from build123d import *

# Parameters (mm, degrees)
PAD_DEPTH = 15
FILLET_R  = 1


with BuildPart() as part:
    # Sketch → Pad (new body)
    with BuildSketch(Plane.XY):
        with BuildLine():
            ThreePointArc((17.433407, 1.525225), (-17.5, 0), (17.433407, -1.525225))
            Line((17.433407, -1.525225), (25.402965, -2.222471))
            ThreePointArc((25.402965, 2.222471), (-25.5, 0), (25.402965, -2.222471))
            Line((17.433407, 1.525225), (25.402965, 2.222471))
        make_face()
    extrude(amount=PAD_DEPTH)

    # Fillet
    fillet_edges = [part.edges().sort_by_distance(p)[0] for p in [
        (17.433407, 1.525225, 7.5),
        (17.433407, -1.525225, 7.5),
    ]]
    fillet(fillet_edges, radius=FILLET_R)


solid = part.part
The model under review builds one solid part; all positions refer to its coordinate system, in mm. A direction names the side the tool comes from. Round coordinates to 2 decimals unless told otherwise and drop trailing zeros. Write each loop counter-clockwise with the first axis right and the second up, starting at its lowest first coordinate (ties: lowest second). Pieces come first, ordered by that corner, then holes. Notation, with made-up numbers: (3.25, -12.5) - (32.25, -12.5) arc R36 ccw to (32.25, 21.5) - close; hole circle Ø1 at (47, 87). An arc over 180 degrees is marked (long way). One line per item, written item: value. Start each with the question number.
1. Consider section B-B on z = 6.5. Write out the cut boundary in (x, y).
2. The part is to be moulded in two halves that separate along Y. For faces 3 (the face through (-25.477, 1.09, 7.395)), 4 (the face through (6, -17, 0)), 5 (the face through (21.85, 1.91, 7.4)), say which applies: released by +Y, released by -Y, zero draft, split by the parting line, or undercut.
3. Machinability: for faces 1 (the face through (21.85, -1.91, 7.4)), 2 (the face through (6, -17, 15)), which of the approach directions +Z, -Z, +X, -X, +Y, -Y give a long, thin tool a straight path to every point of the face, cutting with its end or side? Answer none if there is none.
4. Consider section A-A on x = 0. Write out the cut boundary in (y, z), and give its area (3 significant figures).
5. To check wall thickness, follow L1, parallel to Y at x = 0, z = 5.75; L2, parallel to Y at x = 3.5, z = 8; L3, parallel to X at y = 0, z = 10. State the ranges of each line that lie inside material, in increasing order. Write a range as from..to.
6. Clearance check with flat-ended pins moving along their axes: P1, Ø1, axis at x = -4.5, z = 12.5, coming from the +Y side; P2, Ø1, axis at x = 9.5, z = 1.5, coming from the +Y side; P3, Ø5, axis at y = 19, z = 7, coming from the -X side. State where each tip first meets the part, or that it passes through.
7. Consider section C-C on x = 13. Write out the cut boundary in (y, z), and give its area (3 significant figures).
8. Consider section D-D on y = 0. Write out the cut boundary in (x, z), and give its area (3 significant figures).
Checks:
1. outline: (17.33, -2.47) arc R17.5 cw (long way) to (17.33, 2.47) arc R1 ccw to (18.4, 1.61) - (25.4, 2.22) arc R25.5 ccw (long way) to (25.4, -2.22) - (18.4, -1.61) arc R1 ccw to start
2. face 3: split by the parting line
2. face 4: zero draft
2. face 5: undercut
3. face 1: +Z, -Z, +X
3. face 2: +Z, +X, -X, +Y, -Y
4. outline: (-25.5, 0) - (-17.5, 0) - (-17.5, 15) - (-25.5, 15) - close; (17.5, 0) - (25.5, 0) - (25.5, 15) - (17.5, 15) - close
4. area: 240 mm^2
5. L1: y = -25.5..-17.5, 17.5..25.5
5. L2: y = -25.26..-17.15, 17.15..25.26
5. L3: x = -25.5..-17.5
6. P1: stops at y = 25.18
6. P2: stops at y = 23.86
6. P3: stops at x = -19.44
7. outline: (-21.94, 0) - (-11.72, 0) - (-11.72, 15) - (-21.94, 15) - close; (11.72, 0) - (21.94, 0) - (21.94, 15) - (11.72, 15) - close
7. area: 307 mm^2
8. outline: (-25.5, 0) - (-17.5, 0) - (-17.5, 15) - (-25.5, 15) - close
8. area: 120 mm^2
